Verification items for the finished model (mm, model axes). Face numbers are marked on the shaded views. A direction names the side the tool comes from. Coordinates: 2 decimals unless noted, no trailing zeros. Order: outer loops, then holes, each group sorted by start corner. A loop starts at its lowest first (then second) coordinate and runs counter-clockwise, first axis right, second up. Notation, with made-up numbers: M -13,6.25 L 22,6.25 A20 cw 22,31.25 Z; hole C -27,-16.75 d10. An arc over 180 degrees is marked long. Use one line per item in the form item = value. Start each with the question number.
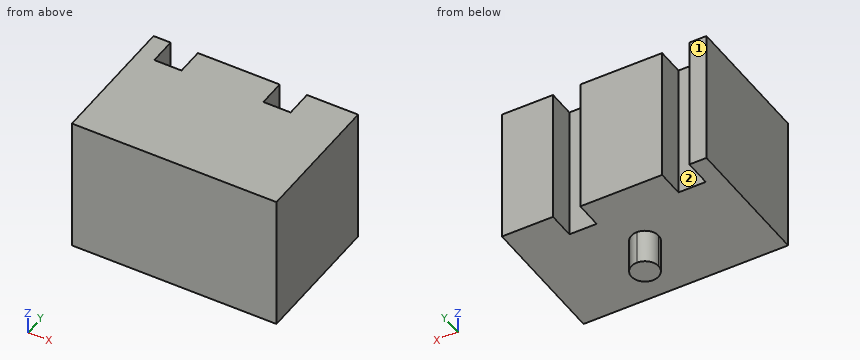
```python
from build123d import *

# Parameters (mm, degrees)
F0_W     = 30
F0_H     = 20
F1_DEPTH = 20
F2_W     = 4
F2_H     = 4
F3_DEPTH = 20.001
F5_DEPTH = 5


with BuildPart() as f1:
    # F0 (on Top) → F1 (new body)
    with BuildSketch(Plane.XY):
        with Locations((15, 10)):
            Rectangle(F0_W, F0_H)
    extrude(amount=F1_DEPTH)

    # F2 (on face) → F3 (cut, through all)
    with BuildSketch(Plane.XY.offset(20)):
        with Locations((4.5, 18)):
            Rectangle(F2_W, F2_H)
        with Locations((20.5, 18)):
            Rectangle(F2_W, F2_H)
    extrude(amount=-F3_DEPTH, mode=Mode.SUBTRACT)

    # F4 (on face) → F5 (join)
    with BuildSketch(Plane(origin=(0, 0, 0), x_dir=(1, 0, 0), z_dir=(0, 0, -1))):
        with BuildLine():
            ThreePointArc((15, -8), (13.585786, -8.585786), (13, -10))
            Line((13, -10), (15, -10))
            Line((15, -10), (15, -8))
        make_face()
        with BuildLine():
            Line((15, -10), (13, -10))
            ThreePointArc((13, -10), (13.585786, -11.414214), (15, -12))
            Line((15, -12), (15, -10))
        make_face()
        with BuildLine():
            Line((15, -8), (15, -10))
            Line((15, -10), (17, -10))
            ThreePointArc((17, -10), (16.414214, -8.585786), (15, -8))
        make_face()
        with BuildLine():
            Line((17, -10), (15, -10))
            Line((15, -10), (15, -12))
            ThreePointArc((15, -12), (16.414214, -11.414214), (17, -10))
        make_face()
    extrude(amount=F5_DEPTH)


solid = f1.part
```
1. Cross-section at B-B on z = 7.5. Enter the section's corners in (x, y).
2. Depth check by flat-ended pin: P1, Ø3, axis at y = 3.5, z = 9.5, coming from the -X side; P2, Ø1.5, axis at x = 15.5, y = 3.5, coming from the -Z side. Enter the tip coordinate at first touch or a pass-through.
3. Cross-section at A-A on y = 18.25. Enter the section's corners in (x, z), and give its area (3 significant figures).
4. Cross-section at C-C on x = 25.25. Enter the section's corners in (y, z), and give its area (3 significant figures).
5. Cross-section at D-D on y = 11. Enter the section's corners in (x, z), and give its area (3 significant figures).
6. Material ranges on line 1 along X through (y, z) = (18, 6.5); line 2 along Y through (x, z) = (6.25, 8.25); line 3 along Z through (x, y) = (11.5, 12.75), recorded low to high.
7. Tool access check on the marked faces 1 and 2. Record the directions out of +Z, -Z, +X, -X, +Y, -Y that give a thin tool (end or side, any length) a straight path to the whole face; none if there is none.
Final values:
q1.outline = M 0,0 L 30,0 L 30,20 L 22.5,20 L 22.5,16 L 18.5,16 L 18.5,20 L 6.5,20 L 6.5,16 L 2.5,16 L 2.5,20 L 0,20 Z
q2.P1 = 0
q2.P2 = 0
q3.outline = M 0,0 L 2.5,0 L 2.5,20 L 0,20 Z; M 6.5,0 L 18.5,0 L 18.5,20 L 6.5,20 Z; M 22.5,0 L 30,0 L 30,20 L 22.5,20 Z
q3.area = 440 mm2
q4.outline = M 0,0 L 20,0 L 20,20 L 0,20 Z
q4.area = 400 mm2
q5.outline = M 0,0 L 13.27,0 L 13.27,-5 L 16.73,-5 L 16.73,0 L 30,0 L 30,20 L 0,20 Z
q5.area = 617 mm2
q6.line_1 = 0 to 2.5, 6.5 to 18.5, 22.5 to 30
q6.line_2 = 0 to 16
q6.line_3 = 0 to 20
q7.face_1 = +Z, -Z, +X, -X, +Y
q7.face_2 = +Z, -Z, +Y
